from build123d import *

# Parameters (mm, degrees)
F1_DEPTH = 15


with BuildPart() as f1:
    # F0 (on Top) → F1 (new body)
    with BuildSketch(Plane.XY):
        with BuildLine():
            Line((0, 40), (0, -43))
            Line((0, -43), (3, -43))
            Line((3, -43), (3, -7))
            ThreePointArc((3, -7), (4.171573, -4.171573), (7, -3))
            Line((7, -3), (63, -3))
            ThreePointArc((63, -3), (65.828427, -4.171573), (67, -7))
            Line((67, -7), (67, -48))
            ThreePointArc((67, -48), (65.828427, -50.828427), (63, -52))
            Line((63, -52), (52.673683, -52))
            Line((52.673683, -52), (52.673683, -55))
            Line((52.673683, -55), (65, -55))
            ThreePointArc((65, -55), (68.535534, -53.535534), (70, -50))
            Line((70, -50), (70, -5))
            ThreePointArc((70, -5), (68.535534, -1.464466), (65, 0))
            Line((65, 0), (7, 0))
            ThreePointArc((7, 0), (4.171573, 1.171573), (3, 4))
            Line((3, 4), (3, 40))
            Line((3, 40), (0, 40))
        make_face()
    extrude(amount=F1_DEPTH)


solid = f1.part
Work out the finished part from the listing and answer in its coordinate system (mm). A direction names the side the tool comes from. Round coordinates to 2 decimals unless told otherwise and drop trailing zeros. Order: outer loops, then holes, each group sorted by start corner. A loop starts at its lowest first (then second) coordinate and runs counter-clockwise, first axis right, second up. Notation, with made-up numbers: M -8.5,68.25 L 49.5,68.25 A22 cw 49.5,90.25 Z; hole C -37,26 d9. An arc over 180 degrees is marked long. One line per item, written item: value.
Q1. Straight lines are drawn through the part: line 1 (Y direction, x = 61, z = 11); line 2 (X direction, y = -23.5, z = 4.5); line 3 (X direction, y = 21.5, z = 3.25). For each, find the intervals that lie inside material, in ascending order.
Derived:
line 1: -55 to -52, -3 to 0
line 2: 0 to 3, 67 to 70
line 3: 0 to 3
Q2. Determine the mould class of faces 4 (the face through (0, -1, 7)), 5 (the face through (67, -27, 7)), 6 (the face through (3, -25, 7)), 7 (the face through (4.203, 1.141, 7.395)) for opening direction X: released by +X, released by -X, zero draft, split by the parting line, or undercut.
Derived:
face 4: released by -X
face 5: undercut
face 6: undercut
face 7: released by +X
Q3. Find section A-A on y = -13.5. Write down the section's boundary in (x, z), then the cut area to 3 significant figures.
Derived:
outline: M 0,0 L 3,0 L 3,15 L 0,15 Z; M 67,0 L 70,0 L 70,15 L 67,15 Z
area: 90.0 mm²
Q4. Find section B-B on x = 59.5. Write down the section's boundary in (y, z).
Derived:
outline: M -55,0 L -52,0 L -52,15 L -55,15 Z; M -3,0 L 0,0 L 0,15 L -3,15 Z
Q5. Find section D-D on x = 33. Write down the section's boundary in (y, z).
Derived:
outline: M -3,0 L 0,0 L 0,15 L -3,15 Z
Q6. Flat-ended cylindrical pins translate along their axes: pin 1 (5 mm diameter, centred on x = 16.5, z = 10, fed in from -Y); pin 2 (10 mm diameter, centred on x = 60, y = -33, fed in from -Z); pin 3 (0.9 mm diameter, centred on y = -53, z = 5, fed in from -X); pin 4 (7.5 mm diameter, centred on y = 18.5, z = 11, fed in from +X). Find the tip coordinate at first contact, or state that the pin passes through.
Derived:
pin 1: y = -3
pin 2: through
pin 3: x = 52.67
pin 4: x = 3
Q7. Find section C-C on z = 6.5. Write down the section's boundary in (x, y).
Derived:
outline: M 0,-43 L 3,-43 L 3,-7 A4 cw 7,-3 L 63,-3 A4 cw 67,-7 L 67,-48 A4 cw 63,-52 L 52.67,-52 L 52.67,-55 L 65,-55 A5 ccw 70,-50 L 70,-5 A5 ccw 65,0 L 7,0 A4 cw 3,4 L 3,40 L 0,40 Z
Q8. For faces 1 (the face through (35, -3, 7)), 2 (the face through (3, 22, 7)), 3 (the face through (4.141, -4.203, 7.395)), determine the directions among +Z, -Z, +X, -X, +Y, -Y from which every point of the face is accessible in a straight line to the end or side of a thin tool.
Derived:
face 1: +Z, -Z
face 2: +Z, -Z, +X, +Y
face 3: +Z, -Z, -Y
